Verification items for the finished model (mm, model axes). Face numbers are marked on the shaded views. A direction names the side the tool comes from. Round coordinates to 2 decimals unless told otherwise and drop trailing zeros. Write each loop counter-clockwise with the first axis right and the second up, starting at its lowest first coordinate (ties: lowest second). Pieces come first, ordered by that corner, then holes.
from build123d import *

# Parameters (mm, degrees)
F1_DEPTH  = 3
F2_DEPTH  = 273
F3_START  = 267
F3_DEPTH  = 3
F4_W      = 14
F4_H      = 65
F5_DEPTH  = 30
F7_D      = 4
F7_DEPTH  = 8
F7_TIP    = 1.2017212381
F9_D      = 4
F9_DEPTH  = 8
F9_TIP    = 1.2017212381
F4_R      = 5
F10_DEPTH = 6


with BuildPart() as f1:
    # F0 (on Top) → F1 (new body)
    with BuildSketch(Plane.XY):
        with BuildLine():
            Line((-243.5, 2), (-243.5, 0))
            ThreePointArc((-243.5, 0), (0, -248), (243.5, 0))
            Line((243.5, 0), (243.5, 2))
            Line((243.5, 2), (213.5, 2))
            Line((213.5, 2), (213.5, -11))
            Line((213.5, -11), (210.5, -11))
            Line((210.5, -11), (210.5, 37))
            Line((210.5, 37), (-210.5, 37))
            Line((-210.5, 37), (-210.5, -11))
            Line((-210.5, -11), (-213.5, -11))
            Line((-213.5, -11), (-213.5, 2))
            Line((-213.5, 2), (-243.5, 2))
        make_face()
    extrude(amount=F1_DEPTH)

    # F0 (on Top) → F2 (join)
    with BuildSketch(Plane.XY):
        Polygon((248.5, 40), (-248.5, 40), (-248.5, 0), (-243.5, 0), (-243.5, 2), (-213.5, 2), (-213.5, -11), (-210.5, -11), (-210.5, 37), (210.5, 37), (210.5, -11), (213.5, -11), (213.5, 2), (243.5, 2), (243.5, 0), (248.5, 0), align=None)
    extrude(amount=F2_DEPTH)

    # F1_face (on face) → F3 (join)
    with BuildSketch(Plane(origin=(0, -87.9658672931, 3), x_dir=(1, 0, 0), z_dir=(0, 0, 1)).offset(F3_START)):
        with BuildLine():
            Line((-243.5, 89.9658672931), (-243.5, 87.9658672931))
            ThreePointArc((-243.5, 87.9658672931), (0, -160.0341327069), (243.5, 87.9658672931))
            Line((243.5, 87.9658672931), (243.5, 89.9658672931))
            Line((243.5, 89.9658672931), (213.5, 89.9658672931))
            Line((213.5, 89.9658672931), (213.5, 76.9658672931))
            Line((213.5, 76.9658672931), (210.5, 76.9658672931))
            Line((210.5, 76.9658672931), (210.5, 124.9658672931))
            Line((210.5, 124.9658672931), (-210.5, 124.9658672931))
            Line((-210.5, 124.9658672931), (-210.5, 76.9658672931))
            Line((-210.5, 76.9658672931), (-213.5, 76.9658672931))
            Line((-213.5, 76.9658672931), (-213.5, 89.9658672931))
            Line((-213.5, 89.9658672931), (-243.5, 89.9658672931))
        make_face()
    extrude(amount=F3_DEPTH)

    # F4 (on face) → F5 (cut)
    with BuildSketch(Plane.XZ.offset(-2)):
        with Locations((-220.5, 235.5)):
            Rectangle(F4_W, F4_H)
        with Locations((-220.5, 55.5)):
            Rectangle(F4_W, F4_H)
    extrude(amount=-F5_DEPTH, mode=Mode.SUBTRACT)

    # F7 (one way)
    with BuildSketch(Plane.YZ.offset(-210.5)):
        with Locations((12, 257), (12, 227), (12, 37), (12, 67)):
            Circle(F7_D / 2)
    extrude(amount=-F7_DEPTH, mode=Mode.SUBTRACT)
    with Locations(Plane.YZ.offset(-210.5)):
        with Locations((12, 257), (12, 227), (12, 37), (12, 67)):
            with Locations((0, 0, -(F7_DEPTH + F7_TIP / 2))):  # 118° drill point
                Cone(0, F7_D / 2, F7_TIP, mode=Mode.SUBTRACT)

    # F9 (one way)
    with BuildSketch(Plane(origin=(210.5, 0, 0), x_dir=(0, -1, 0), z_dir=(-1, 0, 0))):
        with Locations((4, 155), (4, 143)):
            Circle(F9_D / 2)
    extrude(amount=-F9_DEPTH, mode=Mode.SUBTRACT)
    with Locations(Plane(origin=(210.5, 0, 0), x_dir=(0, -1, 0), z_dir=(-1, 0, 0))):
        with Locations((4, 155), (4, 143)):
            with Locations((0, 0, -(F9_DEPTH + F9_TIP / 2))):  # 118° drill point
                Cone(0, F9_D / 2, F9_TIP, mode=Mode.SUBTRACT)

    # F4 (on face) → F10 (join)
    with BuildSketch(Plane.XZ.offset(-2)):
        with Locations((-233.5, 258)):
            Circle(F4_R)
        with Locations((-233.5, 15)):
            Circle(F4_R)
        with Locations((233.5, 15)):
            Circle(F4_R)
        with Locations((233.5, 258)):
            Circle(F4_R)
    extrude(amount=F10_DEPTH)


solid = f1.part
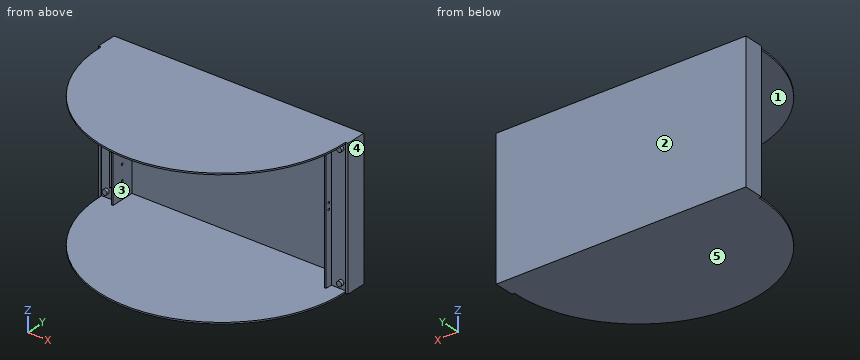
Q1. Material ranges on line 1 along Z through (x, y) = (-131.5, -156.5); line 2 along Z through (x, y) = (-211.6, 12); line 3 along Y through (x, z) = (212.5, 143), recorded low to high.
Recorded:
line 1: z = 0 to 3, 270 to 273
line 2: z = 0 to 35, 39 to 65, 69 to 225, 229 to 255, 259 to 273
line 3: y = -11 to -6, -2 to 40
Q2. Tool access check on the marked faces 1 and 2. Record the directions out of +Z, -Z, +X, -X, +Y, -Y that give a thin tool (end or side, any length) a straight path to the whole face; none if there is none.
Recorded:
face 1: -Y
face 2: +Z, -Z, +X, -X, +Y
Q3. Depth check by flat-ended pin: P1, Ø2.5, axis at y = -4, z = 155, coming from the +X side; P2, Ø10.5, axis at y = -5.5, z = 153, coming from the +X side; P3, Ø12, axis at x = -151, z = 177.5, coming from the -Y side; P4, Ø2, axis at x = 28.5, y = -21, coming from the -Z side. Enter the tip coordinate at first touch or a pass-through.
Recorded:
P1: stops at x = -210.5
P2: stops at x = 213.5
P3: stops at y = 37
P4: stops at z = 0
Q4. Sectioned sample at B-B (y = -45). Enter the section's corners in (x, z), plus the area to 3 significant figures.
Recorded:
outline: (-240.14, 0) - (240.14, 0) - (240.14, 3) - (-240.14, 3) - close; (-240.14, 270) - (240.14, 270) - (240.14, 273) - (-240.14, 273) - close
area: 2,880 mm2
Q5. Sectioned sample at D-D (z = 114.5). Enter the section's corners in (x, y), plus the area to 3 significant figures.
Recorded:
outline: (-248.5, 0) - (-243.5, 0) - (-243.5, 2) - (-213.5, 2) - (-213.5, -11) - (-210.5, -11) - (-210.5, 37) - (210.5, 37) - (210.5, -11) - (213.5, -11) - (213.5, 2) - (243.5, 2) - (243.5, 0) - (248.5, 0) - (248.5, 40) - (-248.5, 40) - close
area: 4,250 mm2
Q6. Sectioned sample at C-C (x = -81). Enter the section's corners in (y, z).
Recorded:
outline: (-234.14, 0) - (40, 0) - (40, 273) - (-234.14, 273) - (-234.14, 270) - (37, 270) - (37, 3) - (-234.14, 3) - close
Q7. Release check for a two-part mould opening along Z. For the marked faces 3, 4 and 5 record: released by +Z, released by -Z, zero draft, split by the parting line, or undercut.
Recorded:
face 3: undercut
face 4: zero draft
face 5: released by -Z
Q8. Sectioned sample at A-A (z = 78.5). Enter the section's corners in (x, y).
Recorded:
outline: (-248.5, 0) - (-243.5, 0) - (-243.5, 2) - (-227.5, 2) - (-227.5, 32) - (-213.5, 32) - (-213.5, -11) - (-210.5, -11) - (-210.5, 37) - (210.5, 37) - (210.5, -11) - (213.5, -11) - (213.5, 2) - (243.5, 2) - (243.5, 0) - (248.5, 0) - (248.5, 40) - (-248.5, 40) - close
